from build123d import *

# Parameters (mm, degrees)
SKETCH1_W           = 38.1
SKETCH1_H           = 25.4
BOSS_EXTRUDE1_DEPTH = 3.175
FILLET1_R           = 12.7
SKETCH2_R           = 2.54
CUT_EXTRUDE1_DEPTH  = 46.900442536


with BuildPart() as part:
    # Sketch1 → Boss-Extrude1 (new body)
    with BuildSketch(Plane.XY):
        with Locations((19.05, 12.7)):
            Rectangle(SKETCH1_W, SKETCH1_H)
    extrude(amount=BOSS_EXTRUDE1_DEPTH)

    # Fillet1
    fillet1_edges = [part.edges().sort_by_distance(p)[0] for p in [
        (38.1, 0, 1.5875),
        (38.1, 25.4, 1.5875),
    ]]
    fillet(fillet1_edges, radius=FILLET1_R - 0.0001)  # a hair under: the kernel refuses the full size

    # Sketch2 → Cut-Extrude1 (cut, through all)
    with BuildSketch(Plane.XY.offset(3.175)):
        with Locations((28.575, 12.7)):
            Circle(SKETCH2_R)
    extrude(amount=-CUT_EXTRUDE1_DEPTH, mode=Mode.SUBTRACT)


solid = part.part
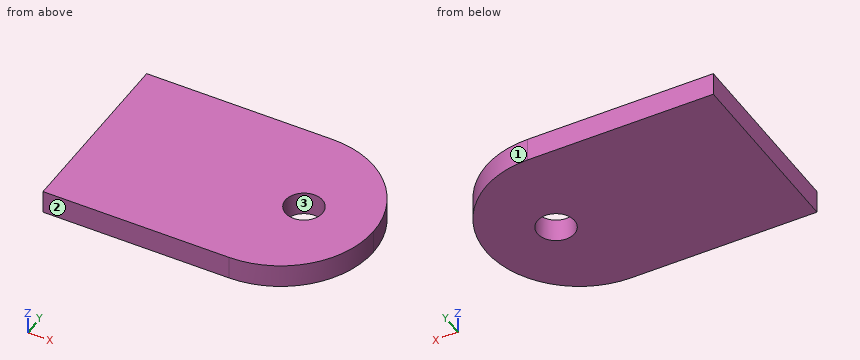
Could you check a few things on this model? Use its own coordinates, in mm. Face numbers are marked on the shaded views. Coordinates: 2 decimals unless noted, no trailing zeros. Write each loop counter-clockwise with the first axis right and the second up, starting at its lowest first coordinate (ties: lowest second). Pieces come first, ordered by that corner, then holes. Notation, with made-up numbers: (72.5, -37.75) - (119.5, -37.75) arc R26 ccw to (119.5, 1.25) - close; hole circle Ø6 at (-10, 15). An arc over 180 degrees is marked (long way). Put each result on its own line as item: value. Start each with the question number.
Q1. I want a section at C-C on y = 17.5. Write out the boundary of the cut face in (x, z) (3 decimals), plus the area to 3 significant figures.
Q2. I want a section at D-D on y = 3.5. Write out the boundary of the cut face in (x, z) (3 decimals).
Q3. Thinking about a two-plate mould opening in X: for the marked faces 1, 2 and 3, which applies, pulls with the +X half, pulls with the -X half, needs draft (parallel to the pull), parting line crosses it, or undercut?
Q4. I want a section at B-B on x = 26.5. Write out the boundary of the cut face in (y, z) (3 decimals).
Q5. Please list where these lines run through material, in increasing order: L1, parallel to X at y = 12.5, z = 1.3; L2, parallel to X at y = 12, z = 3; L3, parallel to Y at x = 29.5, z = 1.65.
Q6. I'm going to push a flat-ended pin straight in: P1, Ø3, axis at x = 28.575, y = 12.7, coming from the +Z side. Where does the tip first touch, or does it pass through?
Checks:
1. outline: (0, 0) - (37.158, 0) - (37.158, 3.175) - (0, 3.175) - close
1. area: 118 mm²
2. outline: (0, 0) - (34.155, 0) - (34.155, 3.175) - (0, 3.175) - close
3. face 1: pulls with the +X half
3. face 2: needs draft
3. face 3: undercut
4. outline: (0.048, 0) - (11.235, 0) - (11.235, 3.175) - (0.048, 3.175) - close; (14.165, 0) - (25.352, 0) - (25.352, 3.175) - (14.165, 3.175) - close
5. L1: 0 to 26.04, 31.11 to 38.1
5. L2: 0 to 26.13, 31.02 to 38.08
5. L3: 0.68 to 10.33, 15.07 to 24.72
6. P1: through
